Verification items for the finished model (mm, model axes). A direction names the side the tool comes from. Round coordinates to 2 decimals unless told otherwise and drop trailing zeros. Order: outer loops, then holes, each group sorted by start corner. A loop starts at its lowest first (then second) coordinate and runs counter-clockwise, first axis right, second up. Notation, with made-up numbers: (-30, 8) -> (18, 8) arc R16 ccw to (18, 34) -> close; hole circle Ø11 at (-36, 4). An arc over 180 degrees is marked (long way). Answer in a Markdown table with one row per item. Add a question column.
Autodesk Inventor part; units mm, degrees
ref_plane "WorkPlane1" through (0, 0, 0) normal (0, 0, 1) x (1, 0, 0)
ref_plane "MSC_PF1" through (0, 0, 0) normal (1, 0, 0) x (0, 1, 0)
ref_plane "MSC_PT1" through (0, 0, 0) normal (0, 0, -1) x (-1, 0, 0)
ref_plane "WorkPlane1" through (0, 0, 0) normal (0, 0, 1) x (1, 0, 0)
sketch "Sketch1" plane through (0, 0, 0) normal (0, 0, 1) x (1, 0, 0)
  point P0 (0, 0)
sketch "Sketch2" plane through (0, 0, 0) normal (0, 0, 1) x (1, 0, 0)
  line L0 (-12, 6.9284) -> (-12, -6.9284)
  line L1 (0, 13.8562) -> (-12, 6.9284)
  line L2 (12, 6.9284) -> (0, 13.8562)
  line L3 (12, -6.9284) -> (12, 6.9284)
  line L4 (0, -13.8562) -> (12, -6.9284)
  line L5 (-12, -6.9284) -> (0, -13.8562)
  circle A0 centre (0, 0) radius 12 construction
  dimension "d1" = 24
  dimension "d29" = 0
  dimension "d30" = 0
extrude "Extrusion1" add sketch "Sketch2" along normal blind 10
sketch "Sketch3" plane through (0, 0, 0) normal (1, 0, 0) x (0, 1, 0)
  line L0 (12, 10) -> (13.9562, 10)
  line L1 (13.9562, 8.8706) -> (12, 10)
  line L2 (13.9562, 10) -> (13.9562, 8.8706)
  line L3 (0, -2) -> (0, 12)
  line L4 (13.8562, 0) -> (13.8562, 10)
  dimension "d25" = 0.1
  dimension "d26" = 0
  dimension "d27" = 60
  dimension "d28" = 12
revolve "Revolution1" cut sketch "Sketch3" angle 360 about axis through (0, 0, -10) along (0, 0, 1)
sketch "Sketch4" plane through (0, 0, 0) normal (1, 0, 0) x (0, 1, 0)
  line L0 (0, -35) -> (0, 0)
  line L1 (-8, -35) -> (0, -35)
  line L2 (-8, 0) -> (-8, -35)
  line L3 (0, 0) -> (-8, 0)
  line L4 (0, -35) -> (0, 0)
  line L5 (-9.6, 0) -> (1.6, 0)
  line L6 (0, -42) -> (0, 7)
  dimension "d18" = 8
  dimension "d20" = 35
  dimension "d33" = 0
  dimension "d34" = 0
revolve "Revolution2" add sketch "Sketch4" angle 360 about axis through (0, 0, -35) along (0, 0, -1)
chamfer "Chamfer1" distance 1 angle 45 1 edges at (0, 8, -35)
fillet "Fillet1" radius 0.6 1 edges at (0, 8, 0)
thread "Thread1"
ref_plane "MSC_PF1" through (0, 0, 0) normal (1, 0, 0) x (0, 1, 0)
ref_plane "MSC_PT1" through (0, 0, 0) normal (0, 0, -1) x (-1, 0, 0)
equation "\"d22\" = 0.5 * PTC"
equation "\"d23\" = 0.5 * PTC"
equation "\"d24\" = r"
equation "\"d1\" = ParS"
equation "\"d6\" = ParK"
equation "\"b\" = NLG - 2 * PTC"
equation "\"d28\" = 0.5 * ParS"
equation "\"d18\" = 0.5 * NND"
equation "\"d20\" = NLG"
equation "\"NND\" = 16"
equation "\"NLG\" = 35"
equation "\"PTC\" = 2"
equation "\"ParK\" = 10"
equation "\"ParS\" = 24"
equation "\"msp_es\" = 0.577367 * ParS"
equation "\"r\" = 0.6"
equation "\"THREADDIA\" = NND"
properties part number "ISO 4018 - M16 x 35" material "Steel"
1) Cross-section at A-A, the plane z = 2. Record the boundary of the cut face in (x, y).
2) Tool access check on faces 1 (the face through (7.81, 1.73, -17.53)), 2 (the face through (5.92, -10.44, 4.93)). Record the directions out of +Z, -Z, +X, -X, +Y, -Y that give a thin tool (end or side, any length) a straight path to the whole face; none if there is none.
3) Cross-section at B-B, the plane z = -9.5. Record the boundary of the cut face in (x, y).
4) Thickness scan on L1, parallel to Z at x = -4.25, y = -10.5; L2, parallel to X at y = 0.25, z = -22; L3, parallel to Y at x = -0.5, z = -33. Record the ranges inside material, lowest first. Write a range as [from, to].
5) Depth check by flat-ended pin: P1, Ø8, axis at x = 6.5, y = 9, coming from the -Z side; P2, Ø3, axis at x = 7.5, z = 2.5, coming from the +Y side; P3, Ø8, axis at y = 3, z = -16, coming from the -X side. Enter the tip coordinate at first touch or a pass-through.
Results below:
| question | item | result |
|---|---|---|
| 1 | outline | (-12, -6.93) -> (0, -13.86) -> (12, -6.93) -> (12, 6.93) -> (0, 13.86) -> (-12, 6.93) -> close |
| 2 | face 1 | -Z |
| 2 | face 2 | +Z, -Z, +X, -Y |
| 3 | outline | circle Ø16 at (0, 0) |
| 4 | L1 | [0, 10] |
| 4 | L2 | [-8, 8] |
| 4 | L3 | [-7.98, 7.98] |
| 5 | P1 | z = -34.9 |
| 5 | P2 | y = 10.39 |
| 5 | P3 | x = -8 |
